The drawing under review shows one solid part. Ordinate dimensions are in mm from its lowest x, y, z. A direction names the side the tool comes from. Coordinates: 2 decimals unless noted, no trailing zeros. Order: outer loops, then holes, each group sorted by start corner. A loop starts at its lowest first (then second) coordinate and runs counter-clockwise, first axis right, second up.
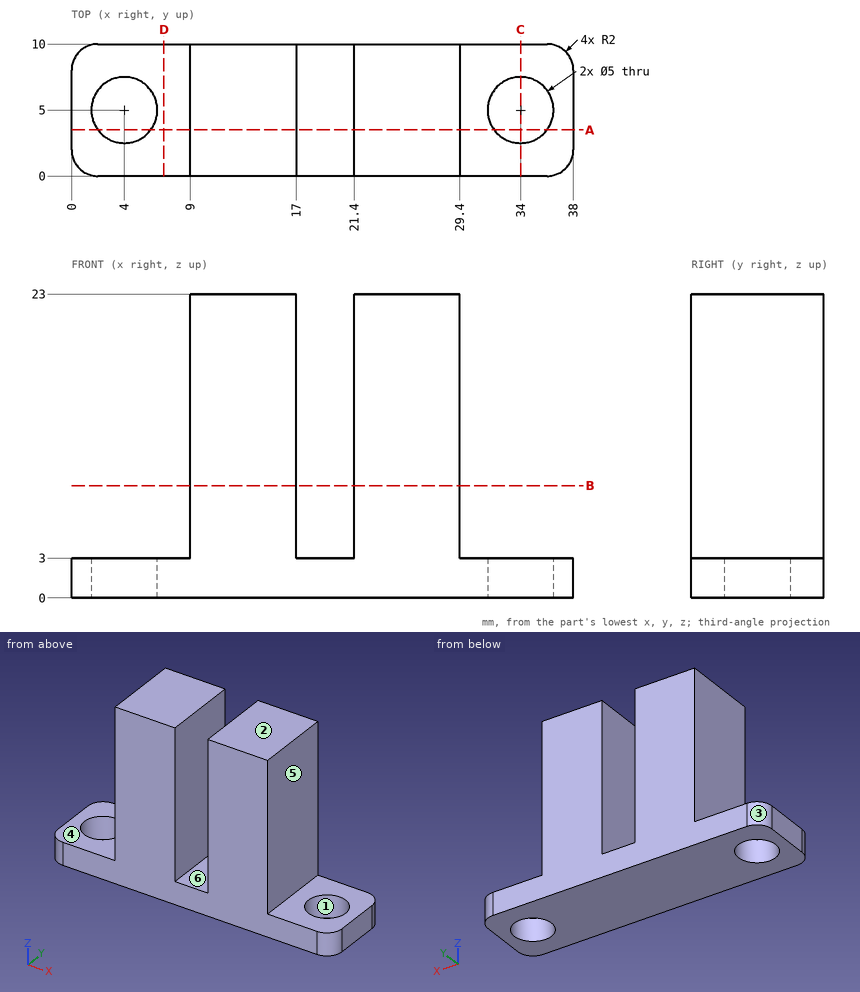
1. Clearance check with flat-ended pins moving along their axes: pin 1 Ø2 at (x, y) = (7, 2) entering from +Z; pin 2 Ø4 at (y, z) = (5.5, 9.5) entering from -X; pin 3 Ø3 at (y, z) = (3.5, 13) entering from +X. State where each tip first meets the part, or that it passes through.
Answer below:
pin 1: stops at z = 3
pin 2: stops at x = 9
pin 3: stops at x = 29.4
2. Take a section at B-B, the plane z = 8.5. Give the boundary of the cut face in (x, y), plus the area to 3 significant figures.
Answer below:
outline: (9, 0) - (17, 0) - (17, 10) - (9, 10) - close; (21.4, 0) - (29.4, 0) - (29.4, 10) - (21.4, 10) - close
area: 160 mm2
3. Take a section at D-D, the plane x = 7. Give the boundary of the cut face in (y, z), plus the area to 3 significant figures.
Answer below:
outline: (0, 0) - (10, 0) - (10, 3) - (0, 3) - close
area: 30.0 mm2
4. To check wall thickness, follow L1, parallel to X at y = 7.25, z = 7.25; L2, parallel to Y at x = 34, z = 1.05; L3, parallel to Z at x = 8, y = 9.25. State the ranges of each line that lie inside material, in increasing order.
Answer below:
L1: x = 9 to 17, 21.4 to 29.4
L2: y = 0 to 2.5, 7.5 to 10
L3: z = 0 to 3
5. Machinability: for the marked faces 4, 5 and 6, which of the approach directions +Z, -Z, +X, -X, +Y, -Y give a long, thin tool a straight path to every point of the face, cutting with its end or side? Answer none if there is none.
Answer below:
face 4: +Z, -X, +Y, -Y
face 5: +Z, +X, +Y, -Y
face 6: +Z, +Y, -Y
6. Take a section at C-C, the plane x = 34. Give the boundary of the cut face in (y, z), plus the area to 3 significant figures.
Answer below:
outline: (0, 0) - (2.5, 0) - (2.5, 3) - (0, 3) - close; (7.5, 0) - (10, 0) - (10, 3) - (7.5, 3) - close
area: 15.0 mm2
7. The part is to be moulded in two halves that separate along X. For the marked faces 1, 2 and 3, say which applies: +X half, -X half, draft (parallel to the pull), parting line (faces both ways), or undercut.
Answer below:
face 1: undercut
face 2: draft
face 3: -X half
8. Take a section at A-A, the plane y = 3.5. Give the boundary of the cut face in (x, z).
Answer below:
outline: (0, 0) - (2, 0) - (2, 3) - (0, 3) - close; (6, 0) - (32, 0) - (32, 3) - (29.4, 3) - (29.4, 23) - (21.4, 23) - (21.4, 3) - (17, 3) - (17, 23) - (9, 23) - (9, 3) - (6, 3) - close; (36, 0) - (38, 0) - (38, 3) - (36, 3) - close
